Source: CAD feature listing. Evaluate the final solid. Frame: model axes, mm. Round coordinates to 2 decimals unless told otherwise and drop trailing zeros. Loops run counter-clockwise (first coordinate to the right, second up) from the corner with the lowest first, then second, coordinate; pieces in that order, holes last.
Item 1: Section query C-C on z = -40. Return loops of the section in (x, y), then the cut area to 3 significant figures.
Item 2: Pull-direction query (X, two-part tool) for faces 1 (the cylindrical face through (-21.115, -9.86, -36.621)), 2 (the flat face through (60, -10, -1)), 3 (the flat face through (-1, 0, 1)); classes: released by +X, released by -X, zero draft, split by the parting line, or undercut.
Item 3: Section query D-D on x = -50. Return loops of the section in (y, z), then the cut area to 3 significant figures.
Item 4: First-contact query: P1, Ø8, axis at x = -17.43, z = -40, coming from the -Y side. Flat tip, straight axial feed; report the tip coordinate or a pass-through.
Item 5: Ray query, L1, parallel to Z at x = -50, y = -9; L2, parallel to X at y = -2.25, z = -37; L3, parallel to X at y = -10, z = -2.5. Return the intervals inside material, ascending.
Item 6: Section query B-B on y = -11.5. Return loops of the section in (x, z), then the cut area to 3 significant figures.
Item 7: Section query A-A on z = 0. Return loops of the section in (x, y), then the cut area to 3 significant figures.
```python
from build123d import *

# Parameters (mm, degrees)
F0_R     = 5
F2_DEPTH = 20


with BuildPart() as f2:
    # F0 (on Front) → F2 (new body)
    with BuildSketch(Plane.XZ):
        with BuildLine():
            Line((29.193788, 50), (-60, 50))
            Line((-60, 50), (-60, -50))
            Line((-60, -50), (60, -50))
            Line((60, -50), (60, 50))
            Line((60, 50), (54.193788, 50))
            ThreePointArc((54.193788, 50), (41.693788, 37.5), (29.193788, 50))
        make_face()
        with Locations((-50, -40)):
            Circle(F0_R, mode=Mode.SUBTRACT)
        with Locations((-17.42937, -40)):
            Circle(F0_R, mode=Mode.SUBTRACT)
        with Locations((-50, 0)):
            Circle(F0_R, mode=Mode.SUBTRACT)
        with Locations((-50.921101, 40)):
            Circle(F0_R, mode=Mode.SUBTRACT)
        with Locations((-18.454628, 40)):
            Circle(F0_R, mode=Mode.SUBTRACT)
    extrude(amount=F2_DEPTH)


solid = f2.part
```
Data:
1. outline: (-60, -20) - (-55, -20) - (-55, 0) - (-60, 0) - close; (-45, -20) - (-22.43, -20) - (-22.43, 0) - (-45, 0) - close; (-12.43, -20) - (60, -20) - (60, 0) - (-12.43, 0) - close
1. area: 2,000 mm2
2. face 1: undercut
2. face 2: released by +X
2. face 3: zero draft
3. outline: (-20, -50) - (0, -50) - (0, -45) - (-20, -45) - close; (-20, -35) - (0, -35) - (0, -5) - (-20, -5) - close; (-20, 5) - (0, 5) - (0, 35.09) - (-20, 35.09) - close; (-20, 44.91) - (0, 44.91) - (0, 50) - (-20, 50) - close
3. area: 1,400 mm2
4. P1: passes through
5. L1: z = -50 to -45, -35 to -5, 5 to 35.09, 44.91 to 50
5. L2: x = -60 to -54, -46 to -21.43, -13.43 to 60
5. L3: x = -60 to -54.33, -45.67 to 60
6. outline: (-60, -50) - (60, -50) - (60, 50) - (54.19, 50) arc R12.5 cw to (29.19, 50) - (-60, 50) - close; hole circle Ø10 at (-50.92, 40); hole circle Ø10 at (-50, -40); hole circle Ø10 at (-50, 0); hole circle Ø10 at (-18.45, 40); hole circle Ø10 at (-17.43, -40)
6. area: 11,400 mm2
7. outline: (-60, -20) - (-55, -20) - (-55, 0) - (-60, 0) - close; (-45, -20) - (60, -20) - (60, 0) - (-45, 0) - close
7. area: 2,200 mm2
